Geometry: see drawing. Coordinates: mm, zero at the bounding-box minimum. Round coordinates to 2 decimals unless told otherwise and drop trailing zeros. Loops run counter-clockwise (first coordinate to the right, second up) from the corner with the lowest first, then second, coordinate; pieces in that order, holes last. Notation, with made-up numbers: (-26, 85) - (1, 85) arc R15 ccw to (1, 108) - close; hole circle Ø7 at (63.5, 0). An arc over 180 degrees is marked (long way). Use CSV: the item, a comma, the result in double quotes. Start each with the question number.
1. Cut plane B-B (x = 0.3). Return loops of the section in (y, z), and give its area (3 significant figures).
2. Cut plane A-A (y = 102). Return loops of the section in (x, z).
3. Pull-direction query (X, two-part tool) for the marked faces 1 and 2; classes: +X half, -X half, draft (parallel to the pull), parting line (faces both ways), or undercut.
4. Cut plane C-C (y = 14). Return loops of the section in (x, z).
5. Material intervals for probe 1 along Y at (x, z) = (0.4, 3.75); probe 2 along Y at (x, z) = (1.45, 2.75); probe 3 along Z at (x, y) = (0.8, 102), sorted ascending. Write a range as from..to.
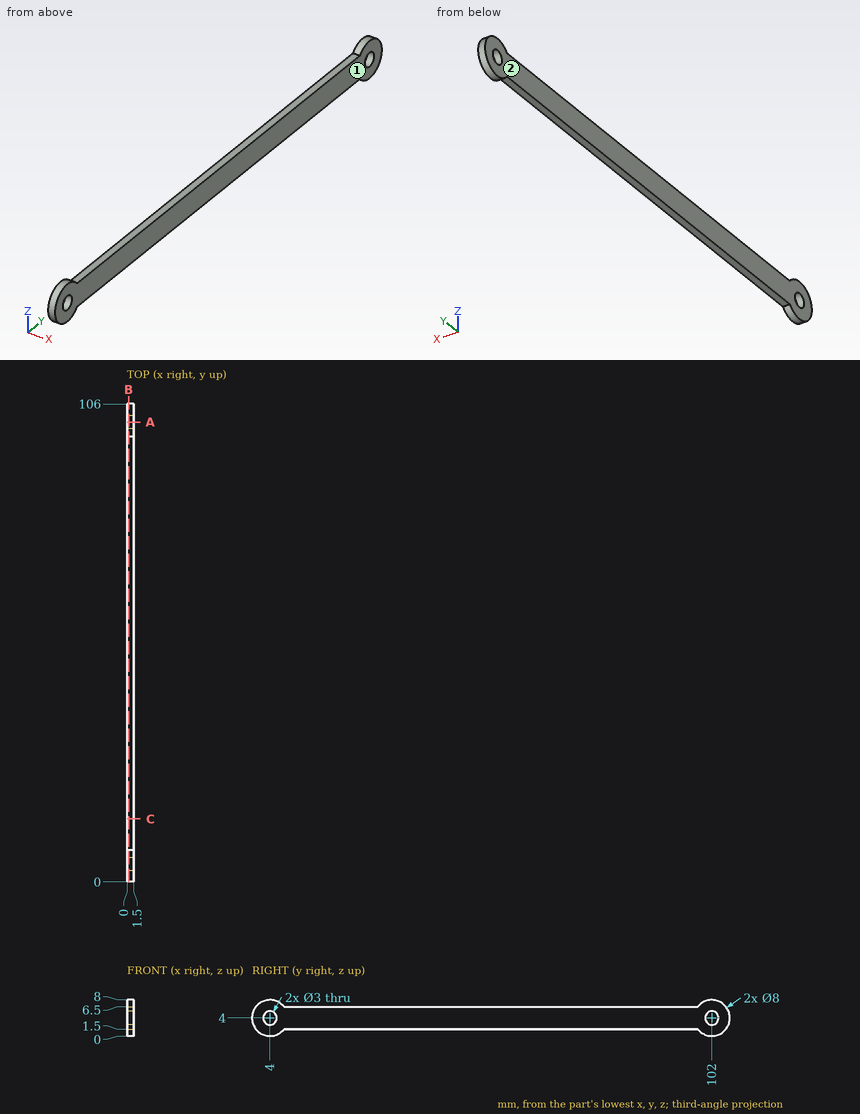
Established:
1,outline,"(7.12, 1.5) - (98.88, 1.5) arc R4 ccw (long way) to (98.88, 6.5) - (7.12, 6.5) arc R4 ccw (long way) to start; hole circle Ø3 at (4, 4); hole circle Ø3 at (102, 4)"
1,area,"539 mm2"
2,outline,"(0, 0) - (1.5, 0) - (1.5, 2.5) - (0, 2.5) - close; (0, 5.5) - (1.5, 5.5) - (1.5, 8) - (0, 8) - close"
3,face 1,"+X half"
3,face 2,"-X half"
4,outline,"(0, 1.5) - (1.5, 1.5) - (1.5, 6.5) - (0, 6.5) - close"
5,probe 1,"y = 0.01..2.52, 5.48..100.52, 103.48..105.99"
5,probe 2,"y = 0.2..3.17, 4.83..101.17, 102.83..105.8"
5,probe 3,"z = 0..2.5, 5.5..8"
